from build123d import *

# Parameters (mm, degrees)
F0_R     = 2
F1_DEPTH = 14.37
F2_DEPTH = 14.37
F3_DEPTH = 7.185
F0_R_2   = 2.05
F4_DEPTH = 14.37


# Not quite as in the source:
# - a feature names something its author has since deleted; it is built from what else it names


with BuildPart() as f1:
    # F0 (on Front) → F1 (new body)
    with BuildSketch(Plane.XZ):
        with Locations((37.2, 2.8)):
            Circle(F0_R)
    extrude(amount=F1_DEPTH)



with BuildPart() as f2:
    # F0 (on Front) → F2 (new body)
    with BuildSketch(Plane.XZ):
        with BuildLine():
            ThreePointArc((5.6, 2.8), (6.4201010127, 0.8201010127), (8.4, 0))
            Line((8.4, 0), (31.6, 0))
            ThreePointArc((31.6, 0), (33.5798989873, 0.8201010127), (34.4, 2.8))
            ThreePointArc((34.4, 2.8), (35.2201010127, 4.7798989873), (37.2, 5.6))
            Line((37.2, 5.6), (37.2, 6.7))
            ThreePointArc((37.2, 6.7), (36.9926506427, 7.3427867688), (36.4487730361, 7.7432436768))
            ThreePointArc((36.4487730361, 7.7432436768), (35.8426991749, 7.6122483799), (35.2574998019, 7.4072435339))
            ThreePointArc((35.2574998019, 7.4072435339), (35.103012566, 6.2352247249), (36.1, 5.6))
            Line((36.1, 5.6), (33.0575369646, 5.6))
            Line((33.0575369646, 5.6), (6.9424630354, 5.6))
            Line((6.9424630354, 5.6), (3.9, 5.6))
            ThreePointArc((3.9, 5.6), (4.896987434, 6.2352247249), (4.7425001981, 7.4072435339))
            ThreePointArc((4.7425001981, 7.4072435339), (4.1573008251, 7.6122483799), (3.5512269639, 7.7432436768))
            ThreePointArc((3.5512269639, 7.7432436768), (3.0073493573, 7.3427867688), (2.8, 6.7))
            Line((2.8, 6.7), (2.8, 5.6))
            ThreePointArc((2.8, 5.6), (4.7798989873, 4.7798989873), (5.6, 2.8))
        make_face()
        with BuildLine():
            ThreePointArc((35.2574998019, 7.4072435339), (34.0261653027, 6.6635182559), (33.0575369646, 5.6))
            Line((33.0575369646, 5.6), (36.1, 5.6))
            ThreePointArc((36.1, 5.6), (35.103012566, 6.2352247249), (35.2574998019, 7.4072435339))
        make_face()
        with BuildLine():
            ThreePointArc((6.9424630354, 5.6), (5.9738346973, 6.6635182559), (4.7425001981, 7.4072435339))
            ThreePointArc((4.7425001981, 7.4072435339), (4.896987434, 6.2352247249), (3.9, 5.6))
            Line((3.9, 5.6), (6.9424630354, 5.6))
        make_face()
    extrude(amount=F2_DEPTH)


with BuildPart() as f1_1:
    add(f1.part)

    add(f2.part)  # F3 merges F2
    # F0 (on Front) → F3 (join)
    with BuildSketch(Plane.XZ):
        with BuildLine():
            ThreePointArc((34.4, 2.8), (35.2201010127, 0.8201010127), (37.2, 0))
            ThreePointArc((37.2, 0), (39.1798989873, 0.8201010127), (40, 2.8))
            ThreePointArc((40, 2.8), (39.1798989873, 4.7798989873), (37.2, 5.6))
            ThreePointArc((37.2, 5.6), (35.2201010127, 4.7798989873), (34.4, 2.8))
        make_face()
        with Locations((37.2, 2.8)):
            Circle(F0_R, mode=Mode.SUBTRACT)
        with BuildLine():
            ThreePointArc((34.4, 2.8), (33.5798989873, 0.8201010127), (31.6, 0))
            Line((31.6, 0), (37.2, 0))
            ThreePointArc((37.2, 0), (35.2201010127, 0.8201010127), (34.4, 2.8))
        make_face()
    extrude(amount=F3_DEPTH)

    # F0 (on Front) → F4 (join)
    with BuildSketch(Plane.XZ):
        with BuildLine():
            ThreePointArc((5.6, 2.8), (4.7798989873, 0.8201010127), (2.8, 0))
            Line((2.8, 0), (8.4, 0))
            ThreePointArc((8.4, 0), (6.4201010127, 0.8201010127), (5.6, 2.8))
        make_face()
        with BuildLine():
            ThreePointArc((2.8, 5.6), (0, 2.8), (2.8, 0))
            ThreePointArc((2.8, 0), (4.7798989873, 0.8201010127), (5.6, 2.8))
            ThreePointArc((5.6, 2.8), (4.7798989873, 4.7798989873), (2.8, 5.6))
        make_face()
        with Locations((2.8, 2.8)):
            Circle(F0_R_2, mode=Mode.SUBTRACT)
    extrude(amount=F4_DEPTH)


solid = f1_1.part
The listing builds one solid part. Answer for the finished solid, in the listing's coordinates (mm). A direction names the side the tool comes from. Give positions to 0.01 mm unless a question says otherwise; leave off trailing zeros. Order: outer loops, then holes, each group sorted by start corner. A loop starts at its lowest first (then second) coordinate and runs counter-clockwise, first axis right, second up. Notation, with made-up numbers: (-6, 20.5) - (34, 20.5) arc R22 ccw to (34, 29.5) - close; hole circle Ø3 at (55.25, -1.5). An arc over 180 degrees is marked (long way). One line per item, written item: value. Start each with the question number.
1) The mould has two halves that part along Z. Classify faces 6 (the face through (39.108, -10.727, 3.401)), 7 (the face through (20, -7, 0)), 8 (the face through (3.013, -7.084, 7.351)), 9 (the face through (20, 0, 3)): released by +Z, released by -Z, zero draft, split by the parting line, or undercut.
2) A tool of negligible diameter and unlimited length cuts with its end or side. For faces 1 (the face through (2.8, -7, 6)), 2 (the face through (20, -7, 5.6)), 3 (the face through (35, -7.185, 2)), 4 (the face through (0.75, -7.08, 2.89)), 5 (the face through (37.2, -7, 6)), from which of +Z, -Z, +X, -X, +Y, -Y can it reach the whole face along a straight path? Write none if from no direction.
3) Given pin 1 Ø5 at (x, y) = (28, -11) entering from +Z; pin 2 Ø1.2 at (y, z) = (-6.5, 6.5) entering from +X; pin 3 Ø4.5 at (x, z) = (2.8, 2.8) entering from -Y, each flat-ended and moving along its own axis, determine where each tip first touches the part or whether it passes through.
4) A cutting plane is placed at C-C on y = -4.75. Give the vertices of the cut face in (x, z), then the cut area to 3 significant figures.
5) A cutting plane is placed at B-B on z = 4.25. Give the vertices of the cut face in (x, y) (1 decimal), then the cut area to 3 significant figures.
6) Find the intervals of material crossed by L1, parallel to Z at x = 18, y = -5.75; L2, parallel to Z at x = 2, y = -9; L3, parallel to X at y = -4, z = 3.5, in increasing order.
7) A cutting plane is placed at D-D on x = 12. Give the vertices of the cut face in (y, z), then the cut area to 3 significant figures.
8) A cutting plane is placed at A-A on y = -9.75. Give the vertices of the cut face in (x, z), then the cut area to 3 significant figures.
Answer sheet:
1. face 6: undercut
1. face 7: released by -Z
1. face 8: released by +Z
1. face 9: zero draft
2. face 1: +Z, -X, +Y, -Y
2. face 2: +Z, +Y, -Y
2. face 3: -Y
2. face 4: +Y, -Y
2. face 5: +Z, +X, +Y, -Y
3. pin 1: stops at z = 5.6
3. pin 2: stops at x = 37.2
3. pin 3: stops at y = -14.37
4. outline: (2.8, 0) - (37.2, 0) arc R2.8 ccw to (37.2, 5.6) - (37.2, 6.7) arc R1.1 ccw to (36.45, 7.74) arc R5 ccw to (33.06, 5.6) - (6.94, 5.6) arc R5 ccw to (3.55, 7.74) arc R1.1 ccw to (2.8, 6.7) - (2.8, 5.6) arc R2.8 ccw to start; hole circle Ø4.1 at (2.8, 2.8)
4. area: 216 mm2
5. outline: (0.4, -14.4) - (1.4, -14.4) - (1.4, 0) - (0.4, 0) - close; (4.2, -14.4) - (34.8, -14.4) - (34.8, -7.2) - (35.8, -7.2) - (35.8, -14.4) - (38.6, -14.4) - (38.6, -7.2) - (39.6, -7.2) - (39.6, 0) - (4.2, 0) - close
5. area: 507 mm2
6. L1: z = 0 to 5.6
6. L2: z = 0.12 to 0.91, 4.69 to 5.48
6. L3: x = 0.09 to 0.87, 4.73 to 39.91
7. outline: (-14.37, 0) - (0, 0) - (0, 5.6) - (-14.37, 5.6) - close
7. area: 80.5 mm2
8. outline: (2.8, 0) - (31.6, 0) arc R2.8 ccw to (34.4, 2.8) arc R2.8 cw to (37.2, 5.6) - (37.2, 6.7) arc R1.1 ccw to (36.45, 7.74) arc R5 ccw to (33.06, 5.6) - (6.94, 5.6) arc R5 ccw to (3.55, 7.74) arc R1.1 ccw to (2.8, 6.7) - (2.8, 5.6) arc R2.8 ccw to start; circle Ø4 at (37.2, 2.8); hole circle Ø4.1 at (2.8, 2.8)
8. area: 201 mm2
